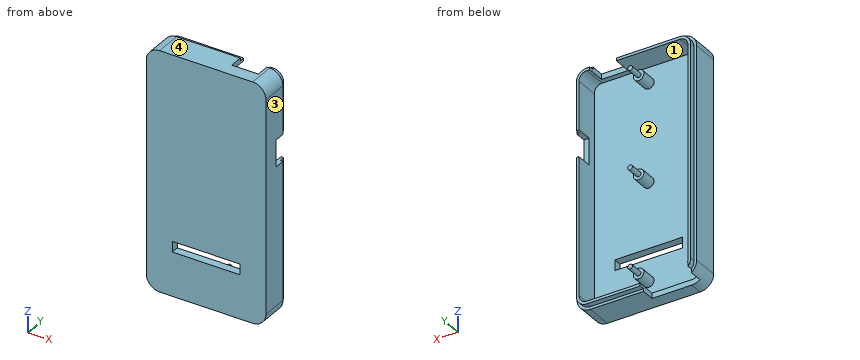
Autodesk Inventor part; units mm, degrees
ref_plane "YZ Plane" through (0, 0, 0) normal (1, 0, 0) x (0, 1, 0)
ref_plane "XZ Plane" through (0, 0, 0) normal (0, 1, 0) x (-1, 0, 0)
ref_plane "XY Plane" through (0, 0, 0) normal (0, 0, 1) x (1, 0, 0)
sketch "Boceto1" plane through (0, 0, 0) normal (0, 1, 0) x (-1, 0, 0)
  line L0 (17.5, 45) -> (-17.5, 45)
  line L1 (-22.5, 40) -> (-22.5, -40)
  line L2 (-17.5, -45) -> (17.5, -45)
  line L3 (22.5, -40) -> (22.5, 40)
  line L4 (22.5, 45) -> (-22.5, -45) construction
  line L5 (-22.5, 45) -> (22.5, -45) construction
  arc A0 (22.5, 40) -> (17.5, 45) centre (17.5, 40) ccw
  arc A1 (-17.5, 45) -> (-22.5, 40) centre (-17.5, 40) ccw
  arc A2 (-22.5, -40) -> (-17.5, -45) centre (-17.5, -40) ccw
  arc A3 (17.5, -45) -> (22.5, -40) centre (17.5, -40) ccw
  point P0 (0, 0)
  dimension "d0" = 45
  dimension "d1" = 90
  dimension "d2" = 5
extrude "Extrusión1" add sketch "Boceto1" along normal blind 10
sketch "Boceto3" plane through (0, 10, 0) normal (0, 1, 0) x (1, 0, 0)
  line L0 (17.5, 43) -> (-17.5, 43)
  arc A0 (-17.5, 43) -> (-20.5, 40) centre (-17.5, 40) ccw
  line L1 (-20.5, 40) -> (-20.5, -40)
  arc A1 (-20.5, -40) -> (-17.5, -43) centre (-17.5, -40) ccw
  line L2 (-17.5, -43) -> (17.5, -43)
  arc A2 (17.5, -43) -> (20.5, -40) centre (17.5, -40) ccw
  line L3 (20.5, -40) -> (20.5, 40)
  arc A3 (20.5, 40) -> (17.5, 43) centre (17.5, 40) ccw
  point P0 (0, 0)
extrude "Extrusión3" cut sketch "Boceto3" against normal blind 7
sketch "Boceto5" plane through (0, 3, 0) normal (0, 1, 0) x (1, 0, 0)
  circle A0 centre (0, 0) radius 2
  dimension "d21" = 4
extrude "Extrusión5" add sketch "Boceto5" along normal blind 6
sketch "Boceto6" plane through (0, 9, 0) normal (0, 1, 0) x (1, 0, 0)
  circle A0 centre (0, 0) radius 2
  circle A1 centre (0, 0) radius 0.9
  dimension "d24" = 1.8
extrude "Extrusión6" add sketch "Boceto6" along normal blind 5 contours A1
sketch "Boceto7" plane through (0, 10, 0) normal (0, 1, 0) x (1, 0, 0)
  line L0 (-20.5, -40) -> (-20.5, 40)
  arc A0 (-17.5, 43) -> (-20.5, 40) centre (-17.5, 40) ccw
  line L1 (-17.5, 43) -> (17.5, 43)
  arc A1 (20.5, 40) -> (17.5, 43) centre (17.5, 40) ccw
  line L2 (20.5, 40) -> (20.5, -40)
  arc A2 (17.5, -43) -> (20.5, -40) centre (17.5, -40) ccw
  line L3 (17.5, -43) -> (-17.5, -43)
  arc A3 (-20.5, -40) -> (-17.5, -43) centre (-17.5, -40) ccw
  arc A4 (17.5, -45) -> (22.5, -40) centre (17.5, -40) ccw
  line L4 (22.5, -40) -> (22.5, 40)
  arc A5 (22.5, 40) -> (17.5, 45) centre (17.5, 40) ccw
  line L5 (17.5, 45) -> (-17.5, 45)
  arc A6 (-17.5, 45) -> (-22.5, 40) centre (-17.5, 40) ccw
  line L6 (-22.5, 40) -> (-22.5, -40)
  arc A7 (-22.5, -40) -> (-17.5, -45) centre (-17.5, -40) ccw
  line L7 (-17.5, -45) -> (17.5, -45)
  line L8 (-17.5, -44) -> (17.5, -44)
  arc A8 (17.5, -44) -> (21.5, -40) centre (17.5, -40) ccw
  line L9 (21.5, -40) -> (21.5, 40)
  arc A9 (21.5, 40) -> (17.5, 44) centre (17.5, 40) ccw
  line L10 (17.5, 44) -> (-17.5, 44)
  arc A10 (-17.5, 44) -> (-21.5, 40) centre (-17.5, 40) ccw
  line L11 (-21.5, 40) -> (-21.5, -40)
  arc A11 (-21.5, -40) -> (-17.5, -44) centre (-17.5, -40) ccw
  point P0 (0, 0)
  dimension "d27" = 1
extrude "Extrusión7" add sketch "Boceto7" along normal blind 2 contours A11 L11 A10 L10 A9 L9 A8 L8
sketch "Boceto8" plane through (0, 3, 0) normal (0, 1, 0) x (1, 0, 0)
  line L0 (17.5, -43) -> (-17.5, -43) construction
  line L1 (0, -43) -> (0, -37) construction
  line L2 (-17.5, 43) -> (17.5, 43) construction
  line L3 (0, 43) -> (0, 37) construction
  circle A0 centre (0, -37) radius 2
  circle A1 centre (0, -37) radius 1.5
  circle A2 centre (0, 37) radius 2
  circle A3 centre (0, 37) radius 1.5
  point P0 (0, 0)
  dimension "d30" = 6
  dimension "d31" = 6
  dimension "d32" = 4
  dimension "d33" = 3
  dimension "d34" = 4
  dimension "d35" = 3
extrude "Extrusión8" add sketch "Boceto8" along normal blind 6 contours A0 | A1 | A2 | A3
sketch "Boceto9" plane through (0, 0, 0) normal (0, -1, 0) x (1, 0, 0)
  line L0 (0, -28.5) -> (23, -28.5) construction
  line L1 (0, -28.5) -> (0, -24.5) construction
  line L2 (12.75, -24.5) -> (-12.75, -24.5)
  line L3 (-12.75, -24.5) -> (-12.75, -28.5)
  line L4 (-12.75, -28.5) -> (12.75, -28.5)
  line L5 (12.75, -28.5) -> (12.75, -24.5)
  line L6 (12.75, -24.5) -> (-12.75, -28.5) construction
  line L7 (-12.75, -24.5) -> (12.75, -28.5) construction
  point P0 (0, 0)
  point P1 (0, -26.5)
  dimension "d38" = 4
  dimension "d39" = 25.5
extrude "Extrusión9" cut sketch "Boceto9" against normal blind 10
sketch "Sketch10" plane through (0, 9, -37) normal (0, 1, 0) x (1, 0, 0)
  circle A0 centre (0, 0) radius 0.9
  point P0 (0, -37)
  dimension "d42" = 1.8
extrude "Extrusion10" add sketch "Sketch10" along normal blind 5
sketch "Sketch11" plane through (0, 9, 37) normal (0, 1, 0) x (1, 0, 0)
  circle A0 centre (0, 0) radius 0.9
  point P0 (0, 37)
  dimension "d45" = 1.8
extrude "Extrusion11" add sketch "Sketch11" along normal blind 5
sketch "Sketch15" plane through (17.5, 0, -45) normal (0, 0, -1) x (-1, 0, 0)
  line L0 (38.0046, 12.0013) -> (20.0046, 12.0013)
  line L1 (20.0046, 12.0013) -> (20.0046, 5.0013)
  line L2 (20.0046, 5.0013) -> (38.0046, 5.0013)
  line L3 (38.0046, 5.0013) -> (38.0046, 12.0013)
  point P0 (17.5, 0)
  dimension "d50" = 18
  dimension "d51" = 7
extrude "Extrusion12" cut sketch "Sketch15" against normal blind 4
sketch "Sketch17" plane through (22.5, 0, 40) normal (1, 0, 0) x (0, 0, -1)
  line L0 (0, 12) -> (80, 12)
  line L1 (18.1121, 12) -> (28.1121, 12)
  line L2 (28.1121, 12) -> (28.1121, 6)
  line L3 (28.1121, 6) -> (18.1121, 6)
  line L4 (18.1121, 6) -> (18.1121, 12)
  point P0 (40, 0)
  dimension "d56" = 10
  dimension "d57" = 6
extrude "Extrusion13" cut sketch "Sketch17" against normal blind 4
sketch "Sketch18" plane through (-17.5, 0, 45) normal (0, 0, 1) x (1, 0, 0)
  line L0 (33.9645, 12) -> (23.9645, 12)
  line L1 (23.9645, 12) -> (23.9645, 5)
  line L2 (23.9645, 5) -> (33.9645, 5)
  line L3 (33.9645, 5) -> (33.9645, 12)
  point P0 (17.5, 0)
  dimension "d60" = 10
  dimension "d61" = 7
extrude "Extrusion14" cut sketch "Sketch18" against normal blind 4
properties part number "Pieza_superior"
The listing builds one solid part. Answer for the finished solid, in the listing's coordinates (mm). Face numbers are marked on the shaded views. Round coordinates to 2 decimals unless told otherwise and drop trailing zeros. Order: outer loops, then holes, each group sorted by start corner. A loop starts at its lowest first (then second) coordinate and runs counter-clockwise, first axis right, second up. Notation, with made-up numbers: (-6.5, 31) -> (16.5, 31) arc R17 cw to (16.5, 48) -> close; hole circle Ø8 at (63.25, 14.5). An arc over 180 degrees is marked (long way). One line per item, written item: value.
Item 1: For a pull along Z with two mould halves and no side action, classify the marked faces 1, 2, 3 and 4 as released by +Z, released by -Z, zero draft, split by the parting line, or undercut.
Taken from the geometry:
face 1: undercut
face 2: undercut
face 3: zero draft
face 4: released by +Z
Item 2: Find section A-A, the plane y = 7.5. State how many separate pieces and enclosed holes the cut face has, then the cut area to 3 significant figures.
Taken from the geometry:
separate pieces: 6
enclosed holes: 0
area: 471 mm2
Item 3: Straight lines are drawn through the part: L1, parallel to X at y = 11, z = 0; L2, parallel to X at y = 4.25, z = 5.5; L3, parallel to Z at x = 7.5, y = 1.75. For each, find the intervals that lie inside material, in ascending order.
Taken from the geometry:
L1: x = -21.5 to -20.5, -0.9 to 0.9, 20.5 to 21.5
L2: x = -22.5 to -20.5, 20.5 to 22.5
L3: z = -45 to -28.5, -24.5 to 45
Item 4: Find section C-C, the plane z = 5.5. Give the vertices of the cut face in (x, y), then the cut area to 3 significant figures.
Taken from the geometry:
outline: (-22.5, 0) -> (22.5, 0) -> (22.5, 10) -> (21.5, 10) -> (21.5, 12) -> (20.5, 12) -> (20.5, 3) -> (-20.5, 3) -> (-20.5, 12) -> (-21.5, 12) -> (-21.5, 10) -> (-22.5, 10) -> close
area: 167 mm2
Item 5: Find section D-D, the plane x = -15. Give the vertices of the cut face in (y, z), then the cut area to 3 significant figures.
Taken from the geometry:
outline: (0, -45) -> (5, -45) -> (5, -43) -> (3, -43) -> (3, 43) -> (12, 43) -> (12, 44) -> (10, 44) -> (10, 45) -> (0, 45) -> close
area: 290 mm2
Item 6: Find section B-B, the plane x = -6. Give the vertices of the cut face in (y, z), then the cut area to 3 significant figures.
Taken from the geometry:
outline: (0, -45) -> (5, -45) -> (5, -43) -> (3, -43) -> (3, -28.5) -> (0, -28.5) -> close; (0, -24.5) -> (3, -24.5) -> (3, 43) -> (12, 43) -> (12, 44) -> (10, 44) -> (10, 45) -> (0, 45) -> close
area: 278 mm2
Item 7: Given P1, Ø1, axis at y = 12, z = -16.5, coming from the -X side; P2, Ø7, axis at x = 12.5, z = -22, coming from the +Y side; P3, Ø1.5, axis at x = 8, y = 11.5, coming from the -Z side, each flat-ended and moving along its own axis, determine where each tip first touches the part or whether it passes through.
Taken from the geometry:
P1: stops at x = -21.5
P2: stops at y = 3
P3: stops at z = -44
